Source: CAD feature listing. Evaluate the final solid. Frame: model axes, mm. A direction names the side the tool comes from. Give positions to 0.01 mm unless a question says otherwise; leave off trailing zeros. Loops run counter-clockwise (first coordinate to the right, second up) from the corner with the lowest first, then second, coordinate; pieces in that order, holes last.
from build123d import *

# Parameters (mm, degrees)
SKETCH_1_R           = 2.75
EXTRUDE_1_DEPTH      = 4.5
EXTRUDE_2_DEPTH      = 22.5
EXTRUDE_2_DEPTH_BACK = 22.5
SKETCH_3_R           = 5
SKETCH_3_R_2         = 3.5
EXTRUDE_3_DEPTH      = 5
SKETCH_4_W           = 10
SKETCH_4_H           = 15
CUT_EXTRUDE_1_DEPTH  = 5
SKETCH_5_W           = 6
SKETCH_5_H           = 2
EXTRUDE_4_DEPTH      = 12.5
SKETCH_6_W           = 6
SKETCH_6_H           = 1.5
EXTRUDE_5_DEPTH      = 14
CUT_EXTRUDE_2_DEPTH  = 20
SKETCH_8_R           = 1.6
CUT_EXTRUDE_3_DEPTH  = 10


with BuildPart() as part:
    # Эскиз1 → Вытянуть1 (new body)
    with BuildSketch(Plane.XY):
        Polygon((-22.5, -16.9), (-37.5, -6.9), (-37.5, 14.1), (37.5, 14.1), (37.5, -6.9), (22.5, -16.9), align=None)
        with Locations((-32.5, 0)):
            Circle(SKETCH_1_R, mode=Mode.SUBTRACT)
        with Locations((32.5, 0)):
            Circle(SKETCH_1_R, mode=Mode.SUBTRACT)
    extrude(amount=EXTRUDE_1_DEPTH)

    # Эскиз2 → Вытянуть2 (add, two sides: drawn at the far end of the back side and taken through both)
    with BuildSketch(Plane(origin=(0, 0, 0), x_dir=(0, 0, -1), z_dir=(1, 0, 0)).offset(-EXTRUDE_2_DEPTH_BACK)):
        Polygon((0, -16.9), (19.60451018, -16.9), (19.60451018, -6.9), (25, -6.9), (25, -3.9), (30, -3.9), (30, 14.1), (0, 14.1), align=None)
    extrude(amount=EXTRUDE_2_DEPTH + EXTRUDE_2_DEPTH_BACK)

    # Эскиз3 → Вытянуть3 (add)
    # profile 1 of 3: a face of its own
    with BuildSketch(Plane(origin=(0, 0, -30), x_dir=(-1, 0, 0), z_dir=(0, 0, -1))):
        with Locations(Location((-15, 5.1, 0), (0, 0, 180))):
            Circle(SKETCH_3_R)
        with Locations((-15, 5.1)):
            Circle(SKETCH_3_R_2, mode=Mode.SUBTRACT)
    # profile 2 of 3: a face of its own
    with BuildSketch(Plane(origin=(0, 0, -30), x_dir=(-1, 0, 0), z_dir=(0, 0, -1))):
        with Locations(Location((15, 5.1, 0), (0, 0, 180))):
            Circle(SKETCH_3_R)
        with Locations((15, 5.1)):
            Circle(SKETCH_3_R_2, mode=Mode.SUBTRACT)
    # profile 3 of 3: a face of its own
    with BuildSketch(Plane(origin=(0, 0, -30), x_dir=(-1, 0, 0), z_dir=(0, 0, -1))):
        with Locations(Location((-0.042603982, 5.1, 0), (0, 0, 180))):
            Circle(SKETCH_3_R)
        with Locations((-0.042603982, 5.1)):
            Circle(SKETCH_3_R_2, mode=Mode.SUBTRACT)
    extrude(amount=EXTRUDE_3_DEPTH)

    # Эскиз4 → Вырез-Вытянуть1 (cut)
    with BuildSketch(Plane.XZ.offset(16.9)):
        with Locations((0, -7.55225509)):
            Rectangle(SKETCH_4_W, SKETCH_4_H)
        with Locations((12.5, -7.55225509)):
            Rectangle(SKETCH_4_W, SKETCH_4_H)
        with Locations((-12.5, -7.55225509)):
            Rectangle(SKETCH_4_W, SKETCH_4_H)
    extrude(amount=-CUT_EXTRUDE_1_DEPTH, mode=Mode.SUBTRACT)

    # Эскиз5 → Вытянуть4 (add)
    with BuildSketch(Plane.XY.offset(4.5)):
        with Locations((-12.5, -2.15)):
            Rectangle(SKETCH_5_W, SKETCH_5_H)
        with Locations((12.5, -2.15)):
            Rectangle(SKETCH_5_W, SKETCH_5_H)
    extrude(amount=EXTRUDE_4_DEPTH)

    # Эскиз6 → Вытянуть5 (add)
    with BuildSketch(Plane(origin=(0, 0, 0), x_dir=(-1, 0, 0), z_dir=(0, 0, -1))):
        with Locations((-25.5, -8.15)):
            Rectangle(SKETCH_6_W, SKETCH_6_H)
        with Locations((-25.5, 9.35)):
            Rectangle(SKETCH_6_W, SKETCH_6_H)
        with Locations((25.5, 9.35)):
            Rectangle(SKETCH_6_W, SKETCH_6_H)
        with Locations((25.5, -8.15)):
            Rectangle(SKETCH_6_W, SKETCH_6_H)
    extrude(amount=EXTRUDE_5_DEPTH)

    # Эскиз7 → Вырез-Вытянуть2 (cut)
    with BuildSketch(Plane.XZ.offset(8.9)):
        Polygon((-22.5, -14), (-28.5, -14), (-28.5, 0), align=None)
        Polygon((22.5, -14), (28.5, 0), (28.5, -14), align=None)
    extrude(amount=-CUT_EXTRUDE_2_DEPTH, mode=Mode.SUBTRACT)

    # Эскиз8 → Вырез-Вытянуть3 (cut)
    with BuildSketch(Plane.XZ.offset(3.15)):
        with Locations((-12.5, 12)):
            Circle(SKETCH_8_R)
        with Locations((12.5, 12)):
            Circle(SKETCH_8_R)
    extrude(amount=-CUT_EXTRUDE_3_DEPTH, mode=Mode.SUBTRACT)


solid = part.part
1) Cut plane C-C (x = 21.5). Return loops of the section in (y, z).
Checks:
outline: (-16.9, -19.6) - (-6.9, -19.6) - (-6.9, -25) - (-3.9, -25) - (-3.9, -30) - (14.1, -30) - (14.1, 4.5) - (-16.9, 4.5) - close
2) Cut plane B-B (x = -32.5). Return loops of the section in (y, z).
Checks:
outline: (-10.23, 0) - (-2.75, 0) - (-2.75, 4.5) - (-10.23, 4.5) - close; (2.75, 0) - (14.1, 0) - (14.1, 4.5) - (2.75, 4.5) - close
3) Pull-direction query (Z, two-part tool) for faces 1 (the flat face through (0, -14, -0.052)), 2 (the flat face through (-25.542, 9.34, -6.902)), 3 (the flat face through (24, 10.1, -4)), 4 (the flat face through (5, -14, -8)); classes: released by +Z, released by -Z, zero draft, split by the parting line, or undercut.
Checks:
face 1: undercut
face 2: released by -Z
face 3: zero draft
face 4: undercut
4) Cut plane A-A (z = 12). Return loops of the section in (x, y).
Checks:
outline: (-15.5, -3.15) - (-14.1, -3.15) - (-14.1, -1.15) - (-15.5, -1.15) - close; (-10.9, -3.15) - (-9.5, -3.15) - (-9.5, -1.15) - (-10.9, -1.15) - close; (9.5, -3.15) - (10.9, -3.15) - (10.9, -1.15) - (9.5, -1.15) - close; (14.1, -3.15) - (15.5, -3.15) - (15.5, -1.15) - (14.1, -1.15) - close
5) Contact query for flat-ended pins moving along their axis: P1, Ø5, axis at x = 12, z = 9, coming from the +Y side; P2, Ø1.5, axis at x = -11, y = -5.5, coming from the -Z side; P3, Ø2, axis at x = 15, y = 4.5, coming from the -Z side; P4, Ø6.5, axis at x = 25, z = -7.5, coming from the +Y side. Output: stop coordinate, or through.
Checks:
P1: stops at y = -1.15
P2: stops at z = -25
P3: stops at z = -30
P4: stops at y = 14.1
6) Ray query, probe 1 along X at (y, z) = (-12, -8); probe 2 along X at (y, z) = (5, -31); probe 3 along Z at (x, y) = (12.5, -1.85). Return the intervals inside material, ascending.
Checks:
probe 1: x = -22.5 to -17.5, -7.5 to -5, 5 to 7.5, 17.5 to 22.5
probe 2: x = -20 to -18.5, -11.5 to -10, -4.96 to -3.46, 3.54 to 5.04, 10 to 11.5, 18.5 to 20
probe 3: z = -30 to 10.4, 13.6 to 17
7) Reachability of faces 5 (the cylindrical face through (19.77, 3.6, -32.47)), 6 (the flat face through (12, -11.9, -7)), 7 (the flat face through (-25, 10.1, -5)), 8 (the flat face through (-25, 8.6, -5)) from +Z, -Z, +X, -X, +Y, -Y: full face, straight path, thin tool, end or side. Return the list, or none.
Checks:
face 5: -Z
face 6: -Y
face 7: -Z, -X, +Y
face 8: -Z, -X
